Here's how the part is built. I have some questions about the finished solid (model axes, mm). Round coordinates to 2 decimals unless told otherwise and drop trailing zeros. Write each loop counter-clockwise with the first axis right and the second up, starting at its lowest first coordinate (ties: lowest second). Pieces come first, ordered by that corner, then holes. Notation, with made-up numbers: M 32,29.5 L 56,29.5 A11 ccw 56,46.5 Z; hole C 58,60 d1. An arc over 180 degrees is marked long. Write item = value, one per line. Start each with the question number.
(1) I want a section at C-C (x = 0). List the corners of the cut face in (y, z) for me, and give its area (3 significant figures).
(2) I want a section at D-D (x = -7.5). Give the number of separate pieces and of enclosed holes in the cut face, and give its area (3 significant figures).
(3) I want a section at A-A (z = 0). List the corners of the cut face in (x, y) for me.
(4) If we mould it in two halves opening along X, with no side actions, what happens to faces 1 (the cylindrical face through (-8.11, 0.5, 14.47)), 2 (the cylindrical face through (16.586, 0.496, -0.208)), 3 (the flat face through (3.1, 0, 10.2))? For each: released by +X, released by -X, zero draft, split by the parting line, or undercut.
(5) I need wall thicknesses on line 1 along X through (y, z) = (0.75, 0); line 2 along X through (y, z) = (0.95, 0.5); line 3 along Z through (x, y) = (-6.5, 0.65). Which ranges of each line are inside material? Lowest first, please.
(6) Will these pins go through, and if not, where does the flat tip stop? pin 1 Ø0.5 at (x, y) = (13.5, 0.5) entering from -Z; pin 2 Ø0.5 at (x, y) = (14, 0.5) entering from +Z.
(7) I want a section at B-B (y = 0.6). List the corners of the cut face in (x, z) for me.
```python
from build123d import *

# Parameters (mm, degrees)
SKETCH_1_R      = 1.6
SKETCH_1_R_2    = 10.2
EXTRUDE_1_DEPTH = 1
CHAMFER_1_SIZE  = 0.2


with BuildPart() as part:
    # 草图1 → 凸台-拉伸1 (new body)
    with BuildSketch(Plane(origin=(0, 0, 0), x_dir=(1, 0, 0), z_dir=(0, 1, 0))):
        with BuildLine():
            ThreePointArc((-2.307521047, -12.996743693), (6.6, -11.43153533), (12.409270728, -4.5))
            Line((12.409270728, -4.5), (15, -4.5))
            ThreePointArc((15, -4.5), (19.5, 0), (15, 4.5))
            Line((15, 4.5), (12.409270728, 4.5))
            ThreePointArc((12.409270728, 4.5), (6.6, 11.43153533), (-2.307521047, 12.996743693))
            Line((-2.307521047, 12.996743693), (-3.602885683, 15.240381057))
            ThreePointArc((-3.602885683, 15.240381057), (-9.75, 16.887495374), (-11.397114317, 10.740381057))
            Line((-11.397114317, 10.740381057), (-10.101749681, 8.496743693))
            ThreePointArc((-10.101749681, 8.496743693), (-13.2, 0), (-10.101749681, -8.496743693))
            Line((-10.101749681, -8.496743693), (-11.397114317, -10.740381057))
            ThreePointArc((-11.397114317, -10.740381057), (-9.75, -16.887495374), (-3.602885683, -15.240381057))
            Line((-3.602885683, -15.240381057), (-2.307521047, -12.996743693))
        make_face()
        with Locations(Location((-7.5, -12.990381057, 0), (0, 0, 270))):
            Circle(SKETCH_1_R, mode=Mode.SUBTRACT)
        with Locations(Location((15, 0, 0), (0, 0, 270))):
            Circle(SKETCH_1_R, mode=Mode.SUBTRACT)
        with Locations(Location((0, 0, 0), (0, 0, 270))):
            Circle(SKETCH_1_R_2, mode=Mode.SUBTRACT)
        with Locations(Location((-7.5, 12.990381057, 0), (0, 0, 270))):
            Circle(SKETCH_1_R, mode=Mode.SUBTRACT)
    extrude(amount=EXTRUDE_1_DEPTH)

    # 倒角1
    chamfer_1_edges = [part.edges().sort_by_distance(p)[0] for p in [
        (19.5, 1, 0),
        (13.704635364, 1, -4.5),
        (15, 0, -1.6),
        (-7.5, 0, 11.390381057),
        (-7.5, 0, -14.590381057),
        (0, 0, -10.2),
        (6.6, 0, 11.43153533),
        (-2.955203365, 0, 14.118562375),
        (-9.75, 0, 16.887495374),
        (6.6, 1, -11.43153533),
        (-10.749431999, 0, 9.618562375),
        (-13.2, 0, 0),
        (-10.749431999, 0, -9.618562375),
        (-9.75, 0, -16.887495374),
        (-2.955203365, 0, -14.118562375),
        (6.6, 0, -11.43153533),
        (13.704635364, 0, -4.5),
        (19.5, 0, 0),
        (-2.955203365, 1, -14.118562375),
        (13.704635364, 0, 4.5),
        (-9.75, 1, -16.887495374),
        (-10.749431999, 1, -9.618562375),
        (-13.2, 1, 0),
        (-10.749431999, 1, 9.618562375),
        (-9.75, 1, 16.887495374),
        (-2.955203365, 1, 14.118562375),
        (6.6, 1, 11.43153533),
        (0, 1, -10.2),
        (-7.5, 1, -14.590381057),
        (-7.5, 1, 11.390381057),
        (15, 1, -1.6),
        (13.704635364, 1, 4.5),
    ]]
    chamfer(chamfer_1_edges, length=CHAMFER_1_SIZE)


solid = part.part
```
Returned:
q1.outline = M 0,-13 L 0.2,-13.2 L 0.8,-13.2 L 1,-13 L 1,-10.4 L 0.8,-10.2 L 0.2,-10.2 L 0,-10.4 Z; M 0,10.4 L 0.2,10.2 L 0.8,10.2 L 1,10.4 L 1,13 L 0.8,13.2 L 0.2,13.2 L 0,13 Z
q1.area = 5.84 mm²
q2.separate_pieces = 4
q2.enclosed_holes = 0
q2.area = 14.4 mm²
q3.outline = M -13.2,0.2 L -13,0 L -10.4,0 L -10.2,0.2 L -10.2,0.8 L -10.4,1 L -13,1 L -13.2,0.8 Z; M 10.2,0.2 L 10.4,0 L 13.2,0 L 13.4,0.2 L 13.4,0.8 L 13.2,1 L 10.4,1 L 10.2,0.8 Z; M 16.6,0.2 L 16.8,0 L 19.3,0 L 19.5,0.2 L 19.5,0.8 L 19.3,1 L 16.8,1 L 16.6,0.8 Z
q4.face_1 = undercut
q4.face_2 = undercut
q4.face_3 = zero draft
q5.line_1 = -13.2 to -10.2, 10.2 to 13.4, 16.6 to 19.5
q5.line_2 = -13.04 to -10.34, 10.34 to 13.32, 16.68 to 19.32
q5.line_3 = -17.38 to -14.24, -11.74 to -7.86, 7.86 to 11.74, 14.24 to 17.38
q6.pin_1 = -4.5
q6.pin_2 = 4.5
q7.outline = M -11.4,-10.74 A4.5 ccw -3.6,-15.24 L -2.31,-13 A13.2 ccw 12.41,-4.5 L 15,-4.5 A4.5 ccw 15,4.5 L 12.41,4.5 A13.2 ccw -2.31,13 L -3.6,15.24 A4.5 ccw -11.4,10.74 L -10.1,8.5 A13.2 ccw -10.1,-8.5 Z; hole C 0,0 d20.4; hole C -7.5,-12.99 d3.2; hole C -7.5,12.99 d3.2; hole C 15,0 d3.2
